```python
from build123d import *

# Parameters (mm, degrees)
SKETCH1_W                 = 20.5
SKETCH1_H                 = 15.5
BOSS_EXTRUDE1_DEPTH       = 8
SHELL1_T                  = 1.5
BOSS_EXTRUDE2_START       = 8
BOSS_EXTRUDE2_OUTLINE_W   = 1.5
BOSS_EXTRUDE2_OUTLINE_H   = 3
BOSS_EXTRUDE2_OUTLINE_W_2 = 3
BOSS_EXTRUDE2_OUTLINE_H_2 = 1.5
BOSS_EXTRUDE2_DEPTH       = 1.5
SKETCH3_W                 = 10
SKETCH3_H                 = 1.5
CUT_EXTRUDE1_DEPTH        = 8
SKETCH4_W                 = 20.5
SKETCH4_H                 = 1.5
BOSS_EXTRUDE3_DEPTH       = 5
FILLET1_R                 = 1
FILLET2_R                 = 1
FILLET3_R                 = 1
SKETCH5_W                 = 1
SKETCH5_H                 = 1.5
CUT_EXTRUDE3_DEPTH        = 8


# Read off the part's stored shape, not the designer's step: Boss-Extrude2
with BuildPart() as part:
    # Sketch1 → Boss-Extrude1 (new body)
    with BuildSketch(Plane(origin=(0, 0, 0), x_dir=(1, 0, 0), z_dir=(0, 1, 0))):
        with Locations((-3.611209964, -0.053380783)):
            Rectangle(SKETCH1_W, SKETCH1_H)
    extrude(amount=BOSS_EXTRUDE1_DEPTH)

    # Shell1
    shell1_openings = [part.faces().sort_by_distance(p)[0] for p in [
        (-3.611209964, 8, 0.053380783),
    ]]
    offset(amount=SHELL1_T, openings=shell1_openings, kind=Kind.INTERSECTION)

    # Boss-Extrude2 outline → Boss-Extrude2 (add)
    with BuildSketch(Plane(origin=(0, 0, 0), x_dir=(1, 0, 0), z_dir=(0, 1, 0)).offset(BOSS_EXTRUDE2_START)):
        with Locations((-14.611209964, -0.053380783)):
            Rectangle(BOSS_EXTRUDE2_OUTLINE_W, BOSS_EXTRUDE2_OUTLINE_H)
        with Locations((-3.611209964, 8.446619217)):
            Rectangle(BOSS_EXTRUDE2_OUTLINE_W_2, BOSS_EXTRUDE2_OUTLINE_H_2)
        with Locations((7.388790036, -0.053380783)):
            Rectangle(BOSS_EXTRUDE2_OUTLINE_W, BOSS_EXTRUDE2_OUTLINE_H)
    extrude(amount=BOSS_EXTRUDE2_DEPTH)

    # Sketch3 → Cut-Extrude1 (cut)
    with BuildSketch(Plane(origin=(0, 8, 0), x_dir=(1, 0, 0), z_dir=(0, 1, 0))):
        with Locations((-8.861209964, -8.553380783)):
            Rectangle(SKETCH3_W, SKETCH3_H)
    extrude(amount=-CUT_EXTRUDE1_DEPTH, mode=Mode.SUBTRACT)

    # Sketch4 → Boss-Extrude3 (add)
    with BuildSketch(Plane(origin=(0, 0, 0), x_dir=(1, 0, 0), z_dir=(0, 1, 0))):
        with Locations((-3.611209964, 6.946619217)):
            Rectangle(SKETCH4_W, SKETCH4_H)
    extrude(amount=BOSS_EXTRUDE3_DEPTH)

    # Fillet1
    fillet1_edges = [part.edges().sort_by_distance(p)[0] for p in [
        (-15.361209964, 9.5, 0.053380783),
    ]]
    fillet(fillet1_edges, radius=FILLET1_R)

    # Fillet2
    fillet2_edges = [part.edges().sort_by_distance(p)[0] for p in [
        (-3.611209964, 9.5, -9.196619217),
        (8.138790036, 9.5, 0.053380783),
    ]]
    fillet(fillet2_edges, radius=FILLET2_R)

    # Fillet3
    fillet3_edges = [part.edges().sort_by_distance(p)[0] for p in [
        (-15.361209964, 3.25, -9.196619217),
        (8.138790036, 3.25, -9.196619217),
        (8.138790036, 3.25, 9.303380783),
        (-15.361209964, 3.25, 9.303380783),
    ]]
    fillet(fillet3_edges, radius=FILLET3_R)

    # Sketch5 → Cut-Extrude3 (cut)
    with BuildSketch(Plane(origin=(0, 8, 0), x_dir=(1, 0, 0), z_dir=(0, 1, 0))):
        with Locations((-3.361209964, -8.553380783)):
            Rectangle(SKETCH5_W, SKETCH5_H)
    extrude(amount=-CUT_EXTRUDE3_DEPTH, mode=Mode.SUBTRACT)


solid = part.part
```
Here's how the part is built. I have some questions about the finished solid (model axes, mm). A direction names the side the tool comes from. Round coordinates to 2 decimals unless told otherwise and drop trailing zeros. Order: outer loops, then holes, each group sorted by start corner. A loop starts at its lowest first (then second) coordinate and runs counter-clockwise, first axis right, second up. Notation, with made-up numbers: M 49.5,6.25 L 55.5,6.25 A17 cw 55.5,26.25 Z; hole C 31.5,15 d7. An arc over 180 degrees is marked long. Use CSV: the item, a comma, the result in double quotes.
1) I'm going to push flat-ended pins straight in: P1, Ø4, axis at x = 3, z = -5, coming from the +Y side; P2, Ø1.3, axis at x = -7, y = 6.5, coming from the +Z side; P3, Ø0.8, axis at x = 7.5, y = 9, coming from the +Z side. Where does each tip first touch, or does it pass through?
Taken from the geometry:
P1,"y = 5"
P2,"z = -7.7"
P3,"z = 1.55"
2) I need wall thicknesses on line 1 along X through (y, z) = (3, 2.25); line 2 along Z through (x, y) = (-0.75, 7.25); line 3 along Z through (x, y) = (3, 3.25). Which ranges of each line are inside material? Lowest first, please. Write a range as [from, to].
Taken from the geometry:
line 1,"[-15.36, -13.86], [6.64, 8.14]"
line 2,"[-9.2, -7.7], [7.8, 9.3]"
line 3,"[-9.2, -6.2], [7.8, 9.3]"
3) I want a section at B-B (z = -7). List the corners of the cut face in (x, y) for me.
Taken from the geometry:
outline,"M -15.36,-1.5 L 8.14,-1.5 L 8.14,8 L 6.64,8 L 6.64,5 L -13.86,5 L -13.86,8 L -15.36,8 Z"
4) I want a section at D-D (x = 0.5). List the corners of the cut face in (y, z) for me, then the cut area to 4 significant figures.
Taken from the geometry:
outline,"M -1.5,-9.2 L 8,-9.2 L 8,-7.7 L 5,-7.7 L 5,-6.2 L 0,-6.2 L 0,7.8 L 8,7.8 L 8,9.3 L -1.5,9.3 Z"
area,"59.25 mm^2"
5) I want a section at A-A (x = -3.5). List the corners of the cut face in (y, z) for me, then the cut area to 3 significant figures.
Taken from the geometry:
outline,"M -1.5,-9.2 L 8.5,-9.2 A1 ccw 9.5,-8.2 L 9.5,-7.7 L 5,-7.7 L 5,-6.2 L 0,-6.2 L 0,9.3 L -1.5,9.3 Z"
area,"49.3 mm^2"
6) If we mould it in two halves opening along X, with no side actions, what happens to faces 1 (the cylindrical face through (7.854, 9.199, 0.032)), 2 (the flat face through (-15, 8, 5)), 3 (the flat face through (-2.861, 4, 9))? For each: pulls with the +X half, pulls with the -X half, needs draft (parallel to the pull), parting line crosses it, or undercut.
Taken from the geometry:
face 1,"pulls with the +X half"
face 2,"needs draft"
face 3,"undercut"
7) On a 3-axis mill with a long thin cutter (end or side, diameter ignored), from which of +Z, -Z, +X, -X, +Y, -Y can I reach the whole of each face in a straight line? I mean faces 4 (the flat face through (-4, 5, -7)), 5 (the flat face through (-13.861, 5, 1)), 6 (the flat face through (5, 8, -8)), 7 (the flat face through (4, 8, 8)), 8 (the flat face through (-15, 9, -1.447)). Say none if no direction works.
Taken from the geometry:
face 4,"+Y"
face 5,"+Z, +Y"
face 6,"-Z, +X, +Y"
face 7,"+Z, +X, -X, +Y"
face 8,"-Z, +X, -X, +Y"
8) I want a section at C-C (y = 0.75). List the corners of the cut face in (x, z) for me, then the cut area to 3 significant figures.
Taken from the geometry:
outline,"M -15.36,-8.2 A1 ccw -14.36,-9.2 L 7.14,-9.2 A1 ccw 8.14,-8.2 L 8.14,8.3 A1 ccw 7.14,9.3 L -2.86,9.3 L -2.86,7.8 L 6.64,7.8 L 6.64,-6.2 L -13.86,-6.2 L -13.86,9.3 L -14.36,9.3 A1 ccw -15.36,8.3 Z"
area,"130 mm^2"
